Geometry check sheet. Reference: the model listing, model coordinates, mm. A direction names the side the tool comes from. Give positions to 0.01 mm unless a question says otherwise; leave off trailing zeros. Order: outer loops, then holes, each group sorted by start corner. A loop starts at its lowest first (then second) coordinate and runs counter-clockwise, first axis right, second up.
from build123d import *

# Parameters (mm, degrees)
SKETCH3_R          = 1.75
CUT_EXTRUDE1_DEPTH = 10


with BuildPart() as part:
    # Sketch1 → Revolve1 (revolve)
    with BuildSketch(Plane(origin=(0, 0, 0), x_dir=(0, 0, -1), z_dir=(1, 0, 0))):
        Polygon((-16, -48.096567582), (-16, -108.096567582), (-25, -108.096567582), (-25, -115.096567582), (-14.25, -115.096567582), (-14.25, -105.096567582), (-6.5, -105.096567582), (-6.5, -58.096567582), (-14.25, -58.096567582), (-14.25, -48.096567582), align=None)
    revolve(axis=Axis((0, 150, 0), (0, -1, 0)))

    # Sketch3 → Cut-Extrude1 (cut)
    with BuildSketch(Plane.XZ.offset(115.096567582)):
        with Locations(Location((0, -21.25, 0), (0, 0, 270))):
            Circle(SKETCH3_R)
        with Locations(Location((-15.0260191, -15.0260191, 0), (0, 0, 270))):
            Circle(SKETCH3_R)
        with Locations(Location((-21.25, 0, 0), (0, 0, 270))):
            Circle(SKETCH3_R)
        with Locations(Location((-15.0260191, 15.0260191, 0), (0, 0, 270))):
            Circle(SKETCH3_R)
        with Locations(Location((0, 21.25, 0), (0, 0, 270))):
            Circle(SKETCH3_R)
        with Locations(Location((15.0260191, 15.0260191, 0), (0, 0, 270))):
            Circle(SKETCH3_R)
        with Locations(Location((21.25, 0, 0), (0, 0, 270))):
            Circle(SKETCH3_R)
        with Locations(Location((15.0260191, -15.0260191, 0), (0, 0, 270))):
            Circle(SKETCH3_R)
    extrude(amount=-CUT_EXTRUDE1_DEPTH, mode=Mode.SUBTRACT)


solid = part.part
Item 1: Gauge pin test, flat ends, axial feed: pin 1 (5.5 mm diameter, centred on x = -15.03, z = -15.03, fed in from +Y); pin 2 (6 mm diameter, centred on x = 9.5, z = 1, fed in from +Y); pin 3 (4 mm diameter, centred on y = -92, z = -1.5, fed in from -X); pin 4 (3 mm diameter, centred on x = 0, z = 21.25, fed in from -Y). Record the tip position at first contact, or that the pin passes through.
Reported:
pin 1: stops at y = -108.1
pin 2: stops at y = -58.1
pin 3: stops at x = -16
pin 4: passes through
Item 2: Sectioned sample at D-D (z = -21.25). Enter the section's corners in (x, y).
Reported:
outline: (-13.17, -115.1) - (-1.75, -115.1) - (-1.75, -108.1) - (-13.17, -108.1) - close; (1.75, -115.1) - (13.17, -115.1) - (13.17, -108.1) - (1.75, -108.1) - close
Item 3: Draft check along Z on faces 1 (the cylindrical face through (-7.509, -111.646, 23.846)), 2 (the cylindrical face through (-16.734, -111.646, -14.647)), 3 (the flat face through (16.3, -108.097, 0.3)). Enter one of: released by +Z, released by -Z, zero draft, split by the parting line, or undercut.
Reported:
face 1: split by the parting line
face 2: undercut
face 3: zero draft
Item 4: Sectioned sample at A-A (x = 0). Enter the section's corners in (y, z).
Reported:
outline: (-115.1, -25) - (-108.1, -25) - (-108.1, -23) - (-115.1, -23) - close; (-115.1, -19.5) - (-108.1, -19.5) - (-108.1, -16) - (-48.1, -16) - (-48.1, -14.25) - (-58.1, -14.25) - (-58.1, -6.5) - (-105.1, -6.5) - (-105.1, -14.25) - (-115.1, -14.25) - close; (-115.1, 14.25) - (-105.1, 14.25) - (-105.1, 6.5) - (-58.1, 6.5) - (-58.1, 14.25) - (-48.1, 14.25) - (-48.1, 16) - (-108.1, 16) - (-108.1, 19.5) - (-115.1, 19.5) - close; (-115.1, 23) - (-108.1, 23) - (-108.1, 25) - (-115.1, 25) - close
Item 5: Sectioned sample at B-B (z = 0). Enter the section's corners in (x, y), and give its area (3 significant figures).
Reported:
outline: (-25, -115.1) - (-23, -115.1) - (-23, -108.1) - (-25, -108.1) - close; (-19.5, -115.1) - (-14.25, -115.1) - (-14.25, -105.1) - (-6.5, -105.1) - (-6.5, -58.1) - (-14.25, -58.1) - (-14.25, -48.1) - (-16, -48.1) - (-16, -108.1) - (-19.5, -108.1) - close; (6.5, -105.1) - (14.25, -105.1) - (14.25, -115.1) - (19.5, -115.1) - (19.5, -108.1) - (16, -108.1) - (16, -48.1) - (14.25, -48.1) - (14.25, -58.1) - (6.5, -58.1) - close; (23, -115.1) - (25, -115.1) - (25, -108.1) - (23, -108.1) - close
area: 1,040 mm2
Item 6: Scan lines: L1, parallel to X at y = -111.5, z = 0; L2, parallel to X at y = -82, z = 0. Record each from-to range of solid material in increasing order.
Reported:
L1: x = -25 to -23, -19.5 to -14.25, 14.25 to 19.5, 23 to 25
L2: x = -16 to -6.5, 6.5 to 16
Item 7: Sectioned sample at C-C (x = -21.25). Enter the section's corners in (y, z).
Reported:
outline: (-115.1, -13.17) - (-108.1, -13.17) - (-108.1, -1.75) - (-115.1, -1.75) - close; (-115.1, 1.75) - (-108.1, 1.75) - (-108.1, 13.17) - (-115.1, 13.17) - close
Item 8: Set-up check for faces 4 (the cylindrical face through (-16.58, -111.65, 14.22)), 5 (the flat face through (3, -58.097, -6)), 6 (the flat face through (3, -105.097, 6)): record each of +Z, -Z, +X, -X, +Y, -Y from which the full face is reachable in a straight line by a thin tool's end or side.
Reported:
face 4: +Y, -Y
face 5: +Y
face 6: -Y
